Design review of the part built by this model. Coordinates are the model's own, in mm. A direction names the side the tool comes from. Round coordinates to 2 decimals unless told otherwise and drop trailing zeros. Order: outer loops, then holes, each group sorted by start corner. A loop starts at its lowest first (then second) coordinate and runs counter-clockwise, first axis right, second up. Notation, with made-up numbers: M -34,-36.5 L 24,-36.5 A15 cw 24,-32.5 Z; hole C -32.75,-39 d5. An arc over 180 degrees is marked long. Write each question's results on one line, items separated by ' | '. Start each with the question number.
Item 1: Take a section at A-A, the plane y = 27.5. Write out the cut boundary in (x, z) (1 decimal), plus the area to 3 significant figures.
Item 2: Clearance check with flat-ended pins moving along their axes: pin 1 (19 mm diameter, centred on y = 15.5, z = 22.5, fed in from -X); pin 2 (2 mm diameter, centred on x = 59.5, z = 50.5, fed in from +Y); pin 3 (10 mm diameter, centred on x = 1.5, z = 51.5, fed in from +Y); pin 4 (11 mm diameter, centred on y = -18, z = 10, fed in from +X) (3 decimals). State where each tip first meets the part, or that it passes through.
Item 3: The part is to be moulded in two halves that separate along X. For faces 4 (the cylindrical face through (31.8, -16.8, 51.8)), 5 (the cylindrical face through (45.8, -0.36, 38.88)), 6 (the flat face through (1, 35, 10.304)), say which applies: +X half, -X half, draft (parallel to the pull), parting line (faces both ways), or undercut.
Item 4: Machinability: for faces 1 (the flat face through (60, 4, 62.704)), 2 (the flat face through (22.225, 17, 19)), 3 (the flat face through (59.5, -0.1, 43.654)), which of the approach directions +Z, -Z, +X, -X, +Y, -Y give a long, thin tool a straight path to every point of the face, cutting with its end or side? Answer none if there is none.
Item 5: Wall thickness on line 1 (Y direction, x = 19.5, z = 52.5); line 2 (Z direction, x = 32, y = 43); line 3 (Y direction, x = 40, z = 58): over which ranges is each line inside the solid? List them lowest first. Write a range as [from, to].
```python
from build123d import *

# Parameters (mm, degrees)
F1_DEPTH = 63.5
F0_W     = 25.2742138386
F0_H     = 19.05
F2_DEPTH = 25.4
F3_DEPTH = 7.9375
F5_R     = 6.35


with BuildPart() as f1:
    # F0 (on Front) → F1 (new body, symmetric)
    with BuildSketch(Plane.XZ):
        Polygon((-41.275, 10.3035005007), (-41.275, -8.7464994993), (41.275, -8.7464994993), (41.275, 10.3035005007), (22.225, 10.3035005007), align=None)
    extrude(amount=F1_DEPTH, both=True)

    # F0 (on Front) → F2 (join, symmetric)
    with BuildSketch(Plane.XZ):
        with Locations((72.9621069193, 53.1787005007)):
            Rectangle(F0_W, F0_H)
        with BuildLine():
            Line((22.225, 10.3035005007), (41.275, 10.3035005007))
            Line((41.275, 10.3035005007), (41.275, 27.7787005007))
            ThreePointArc((41.275, 27.7787005007), (45.9246798487, 39.0040206521), (57.15, 43.6537005007))
            Line((57.15, 43.6537005007), (60.325, 43.6537005007))
            Line((60.325, 43.6537005007), (60.325, 62.7037005007))
            Line((60.325, 62.7037005007), (57.15, 62.7037005007))
            add(Edge.make_bspline(
                [(54.5407420492, 62.6060948613), (55.4032018072, 62.651337728), (56.2728292952, 62.6839548454), (57.15, 62.7037005007)],
                knots=[108.849692603, 108.849692603, 108.849692603, 108.849692603, 111.5045361635, 111.5045361635, 111.5045361635, 111.5045361635], degree=3))
            ThreePointArc((54.5407420492, 62.6060948613), (31.5483988886, 51.5339871867), (22.225, 27.7787005007))
            Line((22.225, 27.7787005007), (22.225, 10.3035005007))
        make_face()
    extrude(amount=F2_DEPTH, both=True)

    # F0 (on Front) → F3 (join, symmetric)
    with BuildSketch(Plane.XZ):
        with BuildLine():
            add(Edge.make_bspline(
                [(-41.275, 10.3035005007), (-4.1324779121, 37.6718258525), (19.1795324712, 60.7511184661), (54.5407420492, 62.6060948613)],
                knots=[0, 0, 0, 0, 108.849692603, 108.849692603, 108.849692603, 108.849692603], degree=3))
            Line((-41.275, 10.3035005007), (22.225, 10.3035005007))
            Line((22.225, 10.3035005007), (22.225, 27.7787005007))
            ThreePointArc((22.225, 27.7787005007), (31.5483988886, 51.5339871867), (54.5407420492, 62.6060948613))
        make_face()
    extrude(amount=F3_DEPTH, both=True)

    # F0 (on Front) → F4 (revolve)
    with BuildSketch(Plane.XZ):
        Polygon((111.125, 67.4535005007), (85.725, 67.4535005007), (85.5992138386, 38.8785005007), (111.125, 38.8785005007), align=None)
    revolve(axis=Axis((85.6621069193, 0, 53.1660005007), (-0.0044019228, 0, -0.9999903115)))

    # F5
    f5_edges = [f1.edges().sort_by_distance(p)[0] for p in [
        (41.275, 63.5, 0.778501),
        (-41.275, 63.5, 0.778501),
        (41.275, -63.5, 0.778501),
        (-41.275, -63.5, 0.778501),
    ]]
    fillet(f5_edges, radius=F5_R)


solid = f1.part
```
Results list:
1) outline: M -41.3,-8.7 L 41.3,-8.7 L 41.3,10.3 L -41.3,10.3 Z | area: 1,570 mm²
2) pin 1: x = -32.65 | pin 2: y = 25.4 | pin 3: through | pin 4: x = 41.275
3) face 4: -X half | face 5: undercut | face 6: draft
4) face 1: +Z, -X | face 2: +Z, -X, +Y | face 3: -Z
5) line 1: [-7.94, 7.94] | line 2: [-8.75, 10.3] | line 3: [-25.4, 25.4]
